from build123d import *

# Parameters (mm, degrees)
F0_W     = 134.62
F0_H     = 12.7
F1_DEPTH = 5.08
F2_W     = 12.7
F2_H     = 12.7
F3_DEPTH = 27.94
F4_W     = 12.7
F4_H     = 12.7
F5_DEPTH = 99.314
F6_R     = 1.5621
F7_DEPTH = 25.4
F8_R     = 1.5621
F9_DEPTH = 25.4


with BuildPart() as f1:
    # F0 (on Front) → F1 (new body)
    with BuildSketch(Plane.XZ):
        Rectangle(F0_W, F0_H)
    extrude(amount=F1_DEPTH)

    # F2 (on face) → F3 (join)
    with BuildSketch(Plane(origin=(0, 0, 0), x_dir=(-1, 0, 0), z_dir=(0, 1, 0))):
        with Locations((-45.16723, 0)):
            Rectangle(F2_W, F2_H)
        with Locations((44.340361, 0)):
            Rectangle(F2_W, F2_H)
    extrude(amount=F3_DEPTH)

    # F4 (on face) → F5 (join)
    with BuildSketch(Plane(origin=(-50.690361, 0, 0), x_dir=(0, -1, 0), z_dir=(-1, 0, 0))):
        with Locations((-21.59, 0)):
            Rectangle(F4_W, F4_H)
    extrude(amount=-F5_DEPTH)

    # F6 (on face) → F7 (cut)
    with BuildSketch(Plane(origin=(0, 0, 0), x_dir=(-1, 0, 0), z_dir=(0, 1, 0))):
        with Locations((-59.575792, 0)):
            Circle(F6_R)
    extrude(amount=-F7_DEPTH, mode=Mode.SUBTRACT)

    # F8 (on face) → F9 (cut)
    with BuildSketch(Plane(origin=(0, 0, 0), x_dir=(-1, 0, 0), z_dir=(0, 1, 0))):
        with Locations((59.000183, 0)):
            Circle(F8_R)
    extrude(amount=-F9_DEPTH, mode=Mode.SUBTRACT)


solid = f1.part
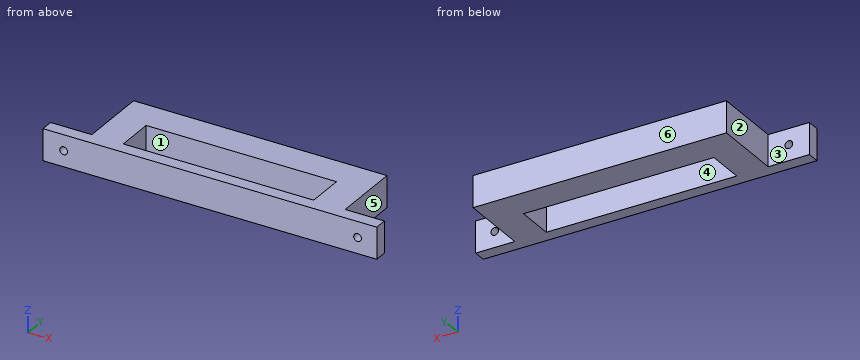
Work out the finished part from the listing and answer in its coordinate system (mm). Face numbers are marked on the shaded views. A direction names the side the tool comes from. Give positions to 0.01 mm unless a question says otherwise; leave off trailing zeros. Write each loop counter-clockwise with the first axis right and the second up, starting at its lowest first coordinate (ties: lowest second). Pieces come first, ordered by that corner, then holes. Notation, with made-up numbers: (51, 37) - (109, 37) arc R18 ccw to (109, 55) - close; hole circle Ø8 at (7.5, -5.75). An arc over 180 degrees is marked (long way). One line per item, written item: value. Start each with the question number.
1. Given pin 1 (12 mm diameter, centred on x = 36.5, y = 8.5, fed in from -Z); pin 2 (3 mm diameter, centred on x = 59.58, z = 0, fed in from -Y); pin 3 (6.5 mm diameter, centred on y = 13, z = 1.5, fed in from +X); pin 4 (4 mm diameter, centred on y = 20.5, z = -2.5, fed in from -X), each flat-ended and moving along its own axis, determine where each tip first touches the part or whether it passes through.
2. Find section A-A (z = 0). Write down the section's boundary in (x, y), then the cut area to 3 significant figures.
3. For the marked faces 5 and 6, determine the directions among +Z, -Z, +X, -X, +Y, -Y from which every point of the face is accessible in a straight line to the end or side of a thin tool.
4. Find section D-D (y = 23). Write down the section's boundary in (x, z), then the cut area to 3 significant figures.
5. For a pull along X with two mould halves and no side action, classify the marked faces 1, 2, 3 and 4 as +X half, -X half, draft (parallel to the pull), parting line (faces both ways), or undercut.
6. Find section C-C (x = -54.5). Write down the section's boundary in (y, z), then the cut area to 3 significant figures.
7. Consider probe 1 along X at (y, z) = (10, 5.5); probe 2 along Y at (x, z) = (30, 1.25); probe 3 along X at (y, z) = (-3, -0.5). Determine where each line is inside the solid, lowest interval first.
8. Find section B-B (x = 35.5). Write down the section's boundary in (y, z).
Geometry results:
1. pin 1: z = -6.35
1. pin 2: through
1. pin 3: x = 51.52
1. pin 4: x = -50.69
2. outline: (-67.31, -5.08) - (-60.56, -5.08) - (-60.56, 0) - (-67.31, 0) - close; (-57.44, -5.08) - (58.01, -5.08) - (58.01, 0) - (51.52, 0) - (51.52, 27.94) - (-50.69, 27.94) - (-50.69, 0) - (-57.44, 0) - close; (61.14, -5.08) - (67.31, -5.08) - (67.31, 0) - (61.14, 0) - close; hole (-37.99, 0) - (38.82, 0) - (38.82, 15.24) - (-37.99, 15.24) - close
2. area: 2,340 mm2
3. face 5: +Z, -Z, +X, +Y
3. face 6: +Z, -Z, +X, -X, +Y
4. outline: (-50.69, -6.35) - (51.52, -6.35) - (51.52, 6.35) - (-50.69, 6.35) - close
4. area: 1,300 mm2
5. face 1: undercut
5. face 2: -X half
5. face 3: draft
5. face 4: undercut
6. outline: (-5.08, -6.35) - (0, -6.35) - (0, 6.35) - (-5.08, 6.35) - close
6. area: 64.5 mm2
7. probe 1: -50.69 to -37.99, 38.82 to 51.52
7. probe 2: -5.08 to 0, 15.24 to 27.94
7. probe 3: -67.31 to -60.48, -57.52 to 58.1, 61.06 to 67.31
8. outline: (-5.08, -6.35) - (0, -6.35) - (0, 6.35) - (-5.08, 6.35) - close; (15.24, -6.35) - (27.94, -6.35) - (27.94, 6.35) - (15.24, 6.35) - close
